Verification items for this drawing (mm, ordinates from the low corner). A direction names the side the tool comes from. Give positions to 0.01 mm unless a question says otherwise; leave off trailing zeros. Order: outer loops, then holes, each group sorted by start corner. A loop starts at its lowest first (then second) coordinate and runs counter-clockwise, first axis right, second up. Notation, with made-up numbers: M 25,76.5 L 65,76.5 A8 cw 65,82.5 Z; hole C 55,15.5 d4. An arc over 180 degrees is marked long. Answer as a JSON object with one key per item and string values.
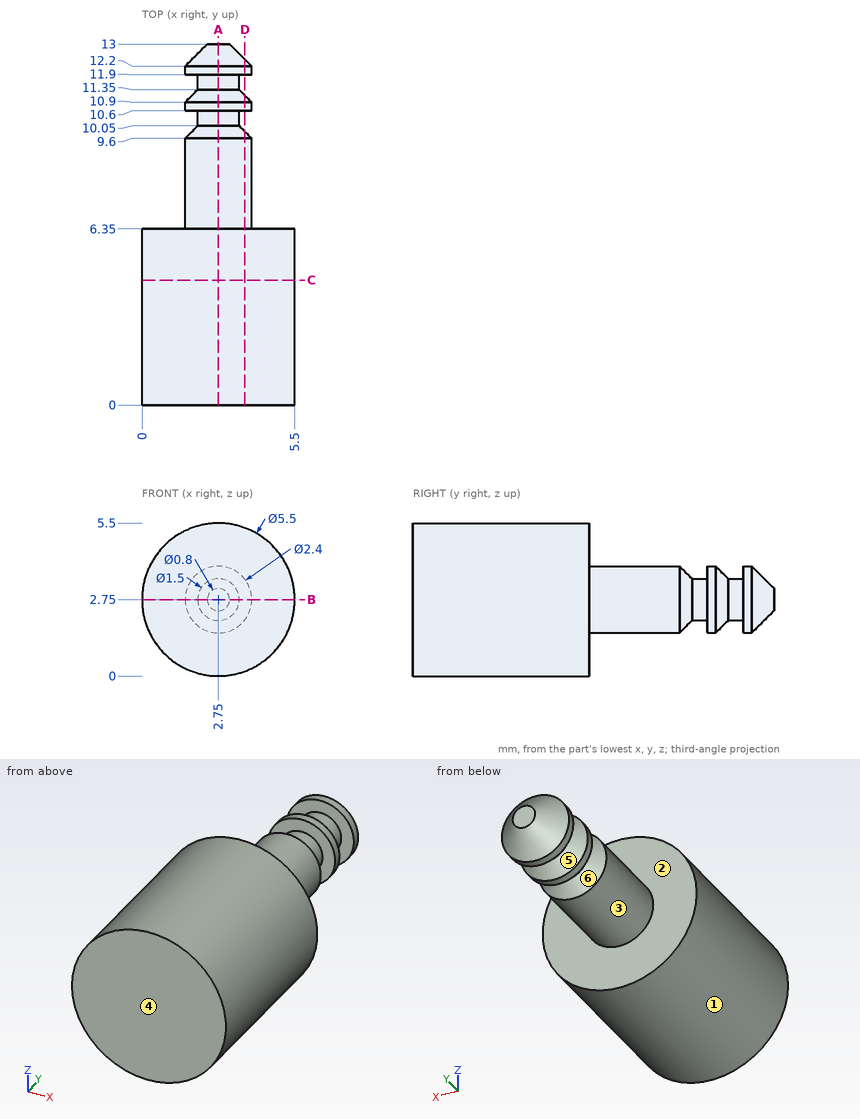
Q1. Section check B-B on z = 2.75. Record the cut outline in (x, y), then the cut area to 4 significant figures.
Resolved:
{"outline": "M 0,0 L 5.5,0 L 5.5,6.35 L 3.95,6.35 L 3.95,9.6 L 3.5,10.05 L 3.5,10.6 L 3.95,10.6 L 3.95,10.9 L 3.5,11.35 L 3.5,11.9 L 3.95,11.9 L 3.95,12.2 L 3.15,13 L 2.35,13 L 1.55,12.2 L 1.55,11.9 L 2,11.9 L 2,11.35 L 1.55,10.9 L 1.55,10.6 L 2,10.6 L 2,10.05 L 1.55,9.6 L 1.55,6.35 L 0,6.35 Z", "area": "48.85 mm²"}
Q2. Tool access check on the marked faces 1 and 2. Record the directions out of +Z, -Z, +X, -X, +Y, -Y that give a thin tool (end or side, any length) a straight path to the whole face; none if there is none.
Resolved:
{"face 1": "+Y, -Y", "face 2": "+Y"}
Q3. Section check C-C on y = 4.5. Record the cut outline in (x, z), then the cut area to 3 significant figures.
Resolved:
{"outline": "C 2.75,2.75 d5.5", "area": "23.8 mm²"}
Q4. Section check D-D on x = 3.7. Count the separate pieces of the cut face and the enclosed holes in it, then the cut area to 3 significant figures.
Resolved:
{"separate pieces": "3", "enclosed holes": "0", "area": "39.1 mm²"}
Q5. Release check for a two-part mould opening along Y. For the marked faces 3, 4, 5 and 6 record: +Y half, -Y half, draft (parallel to the pull), parting line (faces both ways), or undercut.
Resolved:
{"face 3": "draft", "face 4": "-Y half", "face 5": "undercut", "face 6": "undercut"}
Q6. Section check A-A on x = 2.75. Record the cut outline in (y, z).
Resolved:
{"outline": "M 0,0 L 6.35,0 L 6.35,1.55 L 9.6,1.55 L 10.05,2 L 10.6,2 L 10.6,1.55 L 10.9,1.55 L 11.35,2 L 11.9,2 L 11.9,1.55 L 12.2,1.55 L 13,2.35 L 13,3.15 L 12.2,3.95 L 11.9,3.95 L 11.9,3.5 L 11.35,3.5 L 10.9,3.95 L 10.6,3.95 L 10.6,3.5 L 10.05,3.5 L 9.6,3.95 L 6.35,3.95 L 6.35,5.5 L 0,5.5 Z"}
Q7. Material ranges on L1, parallel to Y at x = 4.05, z = 4; L2, parallel to X at y = 12, z = 2.8, recorded low to high.
Resolved:
{"L1": "y = 0 to 6.35", "L2": "x = 1.55 to 3.95"}
Q8. Gauge pin test, flat ends, axial feed: pin 1 Ø1.5 at (x, y) = (4.5, 6) entering from -Z; pin 2 Ø1.5 at (x, y) = (2.5, 9.5) entering from -Z; pin 3 Ø3 at (x, y) = (4, 10.5) entering from +Z. Record the tip position at first contact, or that the pin passes through.
Resolved:
{"pin 1": "stops at z = 0.19", "pin 2": "stops at z = 1.55", "pin 3": "stops at z = 3.95"}
